The model under review builds one solid part; all positions refer to its coordinate system, in mm. Give positions to 0.01 mm unless a question says otherwise; leave off trailing zeros. Order: outer loops, then holes, each group sorted by start corner. A loop starts at its lowest first (then second) coordinate and runs counter-clockwise, first axis right, second up.
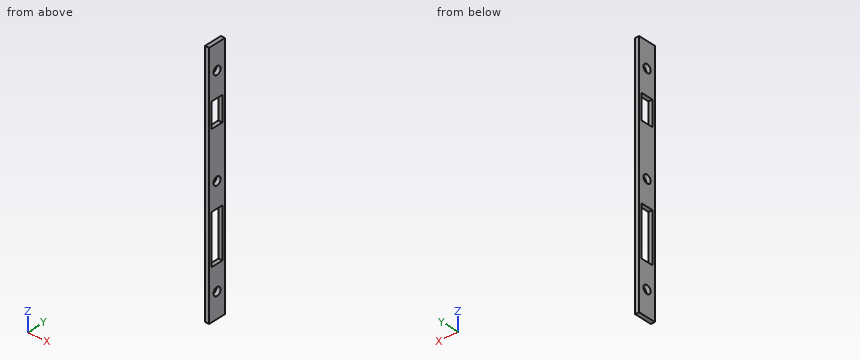
```python
from build123d import *

# Parameters (mm, degrees)
SKETCH1_W           = 300
SKETCH1_H           = 22
BOSS_EXTRUDE1_DEPTH = 5
SKETCH2_R           = 5
SKETCH2_W           = 30
SKETCH2_H           = 15
SKETCH2_W_2         = 60
CUT_EXTRUDE1_DEPTH  = 5


with BuildPart() as part:
    # Sketch1 → Boss-Extrude1 (new body)
    with BuildSketch(Plane(origin=(0, 0, 0), x_dir=(0, 0, -1), z_dir=(1, 0, 0))):
        with Locations((150, 11)):
            Rectangle(SKETCH1_W, SKETCH1_H)
    extrude(amount=BOSS_EXTRUDE1_DEPTH)

    # Sketch2 → Cut-Extrude1 (cut)
    with BuildSketch(Plane(origin=(5, 0, 0), x_dir=(0, 0, -1), z_dir=(1, 0, 0))):
        with Locations((30, 11)):
            Circle(SKETCH2_R)
        with Locations((150, 11)):
            Circle(SKETCH2_R)
        with Locations((270, 11)):
            Circle(SKETCH2_R)
        with Locations((75, 11)):
            Rectangle(SKETCH2_W, SKETCH2_H)
        with Locations((210, 11)):
            Rectangle(SKETCH2_W_2, SKETCH2_H)
    extrude(amount=-CUT_EXTRUDE1_DEPTH, mode=Mode.SUBTRACT)


solid = part.part
```
Item 1: Take a section at C-C (y = 11). Give the boundary of the cut face in (x, z), and give its area (3 significant figures).
Values found:
outline: (0, -300) - (5, -300) - (5, -275) - (0, -275) - close; (0, -265) - (5, -265) - (5, -240) - (0, -240) - close; (0, -180) - (5, -180) - (5, -155) - (0, -155) - close; (0, -145) - (5, -145) - (5, -90) - (0, -90) - close; (0, -60) - (5, -60) - (5, -35) - (0, -35) - close; (0, -25) - (5, -25) - (5, 0) - (0, 0) - close
area: 900 mm2
Item 2: Take a section at B-B (x = 2.25). Give the boundary of the cut face in (y, z).
Values found:
outline: (0, -300) - (22, -300) - (22, 0) - (0, 0) - close; hole (3.5, -240) - (18.5, -240) - (18.5, -180) - (3.5, -180) - close; hole (3.5, -90) - (18.5, -90) - (18.5, -60) - (3.5, -60) - close; hole circle Ø10 at (11, -270); hole circle Ø10 at (11, -150); hole circle Ø10 at (11, -30)
Item 3: Take a section at D-D (z = -150). Give the boundary of the cut face in (x, y), and give its area (3 significant figures).
Values found:
outline: (0, 0) - (5, 0) - (5, 6) - (0, 6) - close; (0, 16) - (5, 16) - (5, 22) - (0, 22) - close
area: 60.0 mm2
Item 4: For line 1 (Z direction, x = 0.45, y = 17.25); line 2 (Z direction, x = 1.5, y = 13.5); line 3 (Y direction, x = 1.65, z = -270), list the stretches that pass through material, from the lowest coordinate up.
Values found:
line 1: z = -300 to -240, -180 to -90, -60 to 0
line 2: z = -300 to -274.33, -265.67 to -240, -180 to -154.33, -145.67 to -90, -60 to -34.33, -25.67 to 0
line 3: y = 0 to 6, 16 to 22
Item 5: Take a section at A-A (z = -224.5). Give the boundary of the cut face in (x, y), and give its area (3 significant figures).
Values found:
outline: (0, 0) - (5, 0) - (5, 3.5) - (0, 3.5) - close; (0, 18.5) - (5, 18.5) - (5, 22) - (0, 22) - close
area: 35.0 mm2
